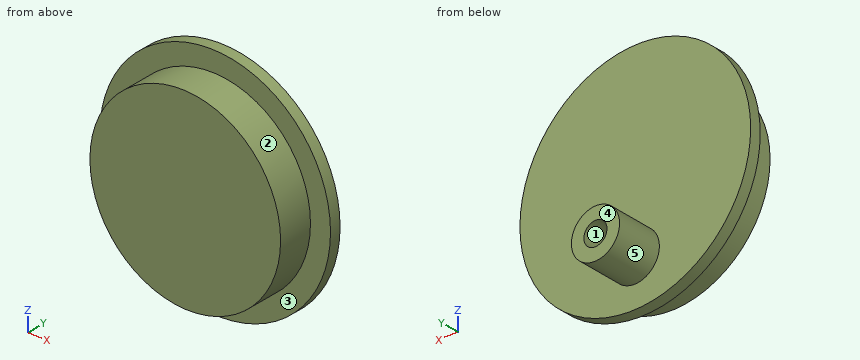
```python
from build123d import *

# Parameters (mm, degrees)
F0_R     = 31.75
F1_DEPTH = 3.048
F2_R     = 26.235323
F3_DEPTH = 9.525
F4_R     = 6.629243
F4_R_2   = 3.175
F5_DEPTH = 12.7


with BuildPart() as f1:
    # F0 (on Front) → F1 (new body)
    with BuildSketch(Plane.XZ):
        Circle(F0_R)
    extrude(amount=F1_DEPTH)

    # F2 (on face) → F3 (join)
    with BuildSketch(Plane.XZ.offset(3.048)):
        Circle(F2_R)
    extrude(amount=F3_DEPTH)

    # F4 (on face) → F5 (join)
    with BuildSketch(Plane(origin=(0, 0, 0), x_dir=(-1, 0, 0), z_dir=(0, 1, 0))):
        with Locations((0, -18.988777)):
            Circle(F4_R)
        with Locations((0, -18.988777)):
            Circle(F4_R_2, mode=Mode.SUBTRACT)
    extrude(amount=F5_DEPTH)


solid = f1.part
```
The listing builds one solid part. Answer for the finished solid, in the listing's coordinates (mm). Face numbers are marked on the shaded views. A direction names the side the tool comes from. Give positions to 0.01 mm unless a question says otherwise; leave off trailing zeros. Write each loop counter-clockwise with the first axis right and the second up, starting at its lowest first coordinate (ties: lowest second). Pieces come first, ordered by that corner, then holes. Notation, with made-up numbers: (67.25, -8) - (78.25, -8) arc R15 ccw to (78.25, 21) - close; hole circle Ø10 at (74.5, 4.25). An arc over 180 degrees is marked (long way). Use one line per item in the form item = value. Start each with the question number.
1) A tool of negligible diameter and unlimited length cuts with its end or side. For the marked faces 4 and 5, from which of +Z, -Z, +X, -X, +Y, -Y can it reach the whole face along a straight path? Write none if from no direction.
2) Find section C-C on y = -7.5. Determine the outline of the cut face in (x, z).
3) Find section B-B on x = 0. Determine the outline of the cut face in (y, z), plus the area to 3 significant figures.
4) The mould has two halves that part along X. Classify the marked faces 1, 2 and 3: pulls with the +X half, pulls with the -X half, needs draft (parallel to the pull), parting line crosses it, or undercut.
5) Find section D-D on z = 19.5. Determine the outline of the cut face in (x, y).
6) Consider line 1 along Z through (x, y) = (0, 9.75); line 2 along Y through (x, z) = (1.5, 10.5); line 3 along Y through (x, z) = (22, 18.5). Determine where each line is inside the solid, lowest interval first. Write a range as from..to.
7) Find section A-A on z = 0. Determine the outline of the cut face in (x, y).
8) Flat-ended cylindrical pins translate along their axes: pin 1 Ø5 at (y, z) = (-9, -8.5) entering from +X; pin 2 Ø6 at (y, z) = (1, 7.5) entering from +X; pin 3 Ø6 at (x, y) = (6, 0.5) entering from +Z. Find the tip coordinate at first contact, or state that the pin passes through.
Geometry results:
q1.face_4 = +Z, -Z, +X, -X, +Y
q1.face_5 = +Y
q2.outline = circle Ø52.47 at (0, 0)
q3.outline = (-12.57, -26.24) - (-3.05, -26.24) - (-3.05, -31.75) - (0, -31.75) - (0, -25.62) - (12.7, -25.62) - (12.7, -22.16) - (0, -22.16) - (0, -15.81) - (12.7, -15.81) - (12.7, -12.36) - (0, -12.36) - (0, 31.75) - (-3.05, 31.75) - (-3.05, 26.24) - (-12.57, 26.24) - close
q3.area = 781 mm2
q4.face_1 = undercut
q4.face_2 = parting line crosses it
q4.face_3 = needs draft
q5.outline = (-25.06, -3.05) - (-17.55, -3.05) - (-17.55, -12.57) - (17.55, -12.57) - (17.55, -3.05) - (25.06, -3.05) - (25.06, 0) - (-25.06, 0) - close
q6.line_1 = -25.62..-22.16, -15.81..-12.36
q6.line_2 = -12.57..0
q6.line_3 = -3.05..0
q7.outline = (-31.75, -3.05) - (-26.24, -3.05) - (-26.24, -12.57) - (26.24, -12.57) - (26.24, -3.05) - (31.75, -3.05) - (31.75, 0) - (-31.75, 0) - close
q8.pin_1 = 25.54
q8.pin_2 = 31.4
q8.pin_3 = 31.6
